from build123d import *

# Parameters (mm, degrees)
CROQUIS1_R              = 1.5
CROQUIS1_R_2            = 2
CROQUIS1_R_3            = 3.5
SALIENTE_EXTRUIR1_DEPTH = 5
REDONDEO1_R             = 5
CROQUIS2_R              = 1.5
CORTAR_EXTRUIR1_DEPTH   = 116.212846506


with BuildPart() as part:
    # Croquis1 → Saliente-Extruir1 (new body)
    with BuildSketch(Plane.XY):
        with BuildLine():
            Line((100, -49), (100, 0))
            Line((100, 0), (100, 5))
            Line((100, 5), (-100, 5))
            Line((-100, 5), (-100, 0))
            Line((-100, 0), (-100, -49))
            ThreePointArc((-100, -49), (-97.656854249, -54.656854249), (-92, -57))
            Line((-92, -57), (92, -57))
            ThreePointArc((92, -57), (97.656854249, -54.656854249), (100, -49))
        make_face()
        with Locations((-35, -45)):
            Circle(CROQUIS1_R, mode=Mode.SUBTRACT)
        with Locations((-15, -45)):
            Circle(CROQUIS1_R, mode=Mode.SUBTRACT)
        with Locations((15, -45)):
            Circle(CROQUIS1_R, mode=Mode.SUBTRACT)
        with Locations((35, -45)):
            Circle(CROQUIS1_R, mode=Mode.SUBTRACT)
        with Locations((-72, -19.25)):
            Circle(CROQUIS1_R_2, mode=Mode.SUBTRACT)
        with Locations((0, -23.25)):
            Circle(CROQUIS1_R_3, mode=Mode.SUBTRACT)
        with Locations((72, -19.25)):
            Circle(CROQUIS1_R_2, mode=Mode.SUBTRACT)
    extrude(amount=SALIENTE_EXTRUIR1_DEPTH)

    # Redondeo1
    redondeo1_edges = [part.edges().sort_by_distance(p)[0] for p in [
        (-100, 5, 2.5),
        (100, 5, 2.5),
    ]]
    fillet(redondeo1_edges, radius=REDONDEO1_R)

    # Croquis2 → Cortar-Extruir1 (cut, through all)
    with BuildSketch(Plane.XY.offset(5)):
        with Locations((0, -14.75)):
            Circle(CROQUIS2_R)
        with Locations((0, -31.75)):
            Circle(CROQUIS2_R)
    extrude(amount=-CORTAR_EXTRUIR1_DEPTH, mode=Mode.SUBTRACT)


solid = part.part
The model under review builds one solid part; all positions refer to its coordinate system, in mm. Coordinates: 2 decimals unless noted, no trailing zeros. Loops run counter-clockwise (first coordinate to the right, second up) from the corner with the lowest first, then second, coordinate; pieces in that order, holes last. Notation, with made-up numbers: M 2,19 L 61,19 A18 ccw 61,40 Z; hole C 72.25,80.25 d9. An arc over 180 degrees is marked long. Put each result on its own line as item: value. Start each with the question number.
Q1. The part is to be moulded in two halves that separate along X. For faces 1 (the cylindrical face through (-98, 4, 3)), 2 (the flat face through (-1, -19, 0)), 3 (the cylindrical face through (-70.092, -18.649, 2.465)), say which applies: +X half, -X half, draft (parallel to the pull), parting line (faces both ways), or undercut.
Q2. Add section A-A (y = -23.25). Write out the cut boundary in (x, z).
Q3. Wall thickness on line 1 (Y direction, x = 0, z = 3.1); line 2 (X direction, y = -32, z = 4.3); line 3 (Y direction, x = 72, z = 2.3): over which ranges is each line inside the solid? List them lowest first.
Q4. Add section B-B (x = 72). Write out the cut boundary in (y, z), and give its area (3 significant figures).
Answers:
1. face 1: -X half
1. face 2: draft
1. face 3: undercut
2. outline: M -100,0 L -3.5,0 L -3.5,5 L -100,5 Z; M 3.5,0 L 100,0 L 100,5 L 3.5,5 Z
3. line 1: y = -57 to -33.25, -30.25 to -26.75, -19.75 to -16.25, -13.25 to 5
3. line 2: x = -100 to -1.48, 1.48 to 100
3. line 3: y = -57 to -21.25, -17.25 to 5
4. outline: M -57,0 L -21.25,0 L -21.25,5 L -57,5 Z; M -17.25,0 L 5,0 L 5,5 L -17.25,5 Z
4. area: 290 mm^2
